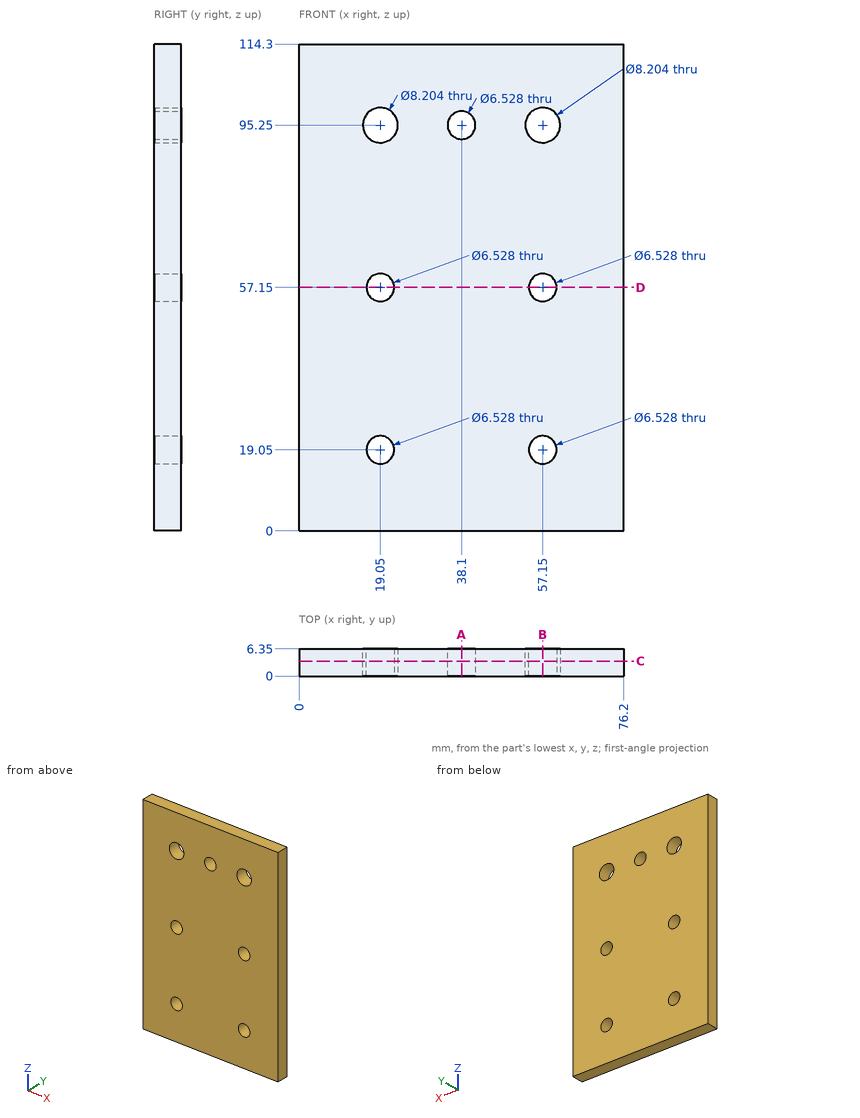
Design review of the part shown in the three views and the two pictorial views. Dimensions are in mm from the part's minimum x, y and z. Give positions to 0.01 mm unless a question says otherwise; leave off trailing zeros. Write each loop counter-clockwise with the first axis right and the second up, starting at its lowest first coordinate (ties: lowest second). Pieces come first, ordered by that corner, then holes. Notation, with made-up numbers: (72.25, 39.25) - (105.25, 39.25) arc R30 cw to (105.25, 64.25) - close; hole circle Ø8 at (88.25, 15). An arc over 180 degrees is marked (long way). Return JSON: item names as keys, results as strings. Group by question number.
(1) We need section A-A, the plane x = 38.1. Give the boundary of the cut face in (y, z), then the cut area to 3 significant figures.
(2) Insertion check: pin 1 (9.5 mm diameter, centred on x = 19.05, z = 95.25, fed in from +Y). The pin has a flat end and moves straight along its axis. Give the tip position at first contact, or say it passes through.
(3) We need section D-D, the plane z = 57.15. Give the boundary of the cut face in (x, y).
(4) We need section C-C, the plane y = 3.5. Give the boundary of the cut face in (x, z).
(5) We need section B-B, the plane x = 57.15. Give the boundary of the cut face in (y, z), then the cut area to 3 significant figures.
(6) To check wall thickness, follow probe 1 along Z at (x, y) = (19.05, 5); probe 2 along X at (y, z) = (1.25, 57.5) (1 decimal); probe 3 along Z at (x, y) = (17, 4.75). State the ranges of each line that lie inside material, in increasing order.
Reported:
{
 "1": {"outline": "(0, 0) - (6.35, 0) - (6.35, 91.99) - (0, 91.99) - close; (0, 98.51) - (6.35, 98.51) - (6.35, 114.3) - (0, 114.3) - close", "area": "684 mm2"},
 "2": {"pin 1": "stops at y = 6.35"},
 "3": {"outline": "(0, 0) - (15.79, 0) - (15.79, 6.35) - (0, 6.35) - close; (22.31, 0) - (53.89, 0) - (53.89, 6.35) - (22.31, 6.35) - close; (60.41, 0) - (76.2, 0) - (76.2, 6.35) - (60.41, 6.35) - close"},
 "4": {"outline": "(0, 0) - (76.2, 0) - (76.2, 114.3) - (0, 114.3) - close; hole circle Ø8.2 at (19.05, 95.25); hole circle Ø6.53 at (19.05, 19.05); hole circle Ø6.53 at (19.05, 57.15); hole circle Ø6.53 at (38.1, 95.25); hole circle Ø8.2 at (57.15, 95.25); hole circle Ø6.53 at (57.15, 19.05); hole circle Ø6.53 at (57.15, 57.15)"},
 "5": {"outline": "(0, 0) - (6.35, 0) - (6.35, 15.79) - (0, 15.79) - close; (0, 22.31) - (6.35, 22.31) - (6.35, 53.89) - (0, 53.89) - close; (0, 60.41) - (6.35, 60.41) - (6.35, 91.15) - (0, 91.15) - close; (0, 99.35) - (6.35, 99.35) - (6.35, 114.3) - (0, 114.3) - close", "area": "591 mm2"},
 "6": {"probe 1": "z = 0 to 15.79, 22.31 to 53.89, 60.41 to 91.15, 99.35 to 114.3", "probe 2": "x = 0 to 15.8, 22.3 to 53.9, 60.4 to 76.2", "probe 3": "z = 0 to 16.51, 21.59 to 54.61, 59.69 to 91.7, 98.8 to 114.3"}
}
